Could you check a few things on this drawing? It's one solid part, dimensions in mm from its lowest x, y, z. A direction names the side the tool comes from. Give positions to 0.01 mm unless a question says otherwise; leave off trailing zeros. Loops run counter-clockwise (first coordinate to the right, second up) from the corner with the lowest first, then second, coordinate; pieces in that order, holes last.
1. Imagine slicing it at D-D (y = 10.25). List the corners of the cut face in (x, z) for me.
2. Imagine slicing it at B-B (x = 3). List the corners of the cut face in (y, z) for me, plus the area to 3 significant figures.
3. Imagine slicing it at C-C (z = 18). List the corners of the cut face in (x, y) for me, plus the area to 3 significant figures.
4. I need wall thicknesses on line 1 along X through (y, z) = (2.9, 3); line 2 along X through (y, z) = (3, 23); line 3 along X through (y, z) = (10.75, 15). Which ranges of each line are inside material? Lowest first, please.
5. Thinking about a two-plate mould opening in X: for the marked faces 1, 2 and 3, which applies, +X half, -X half, draft (parallel to the pull), parting line (faces both ways), or undercut?
6. For P1, Ø5.5, axis at x = 40.5, y = 3, coming from the +Z side; P2, Ø1.8, axis at x = 23, y = 9, coming from the -Z side; P3, Ø3.5, axis at y = 8, z = 28, coming from the +X side, each with a flat end and sliding along its axis, tell me the tip position at first contact or that it passes through.
7. For the marked faces 4 and 5, which set-ups out of +Z, -Z, +X, -X, +Y, -Y let a thin tool reach every point of the face, with its end or its side?
8. Imagine slicing it at A-A (z = 39). List the corners of the cut face in (x, y) for me.
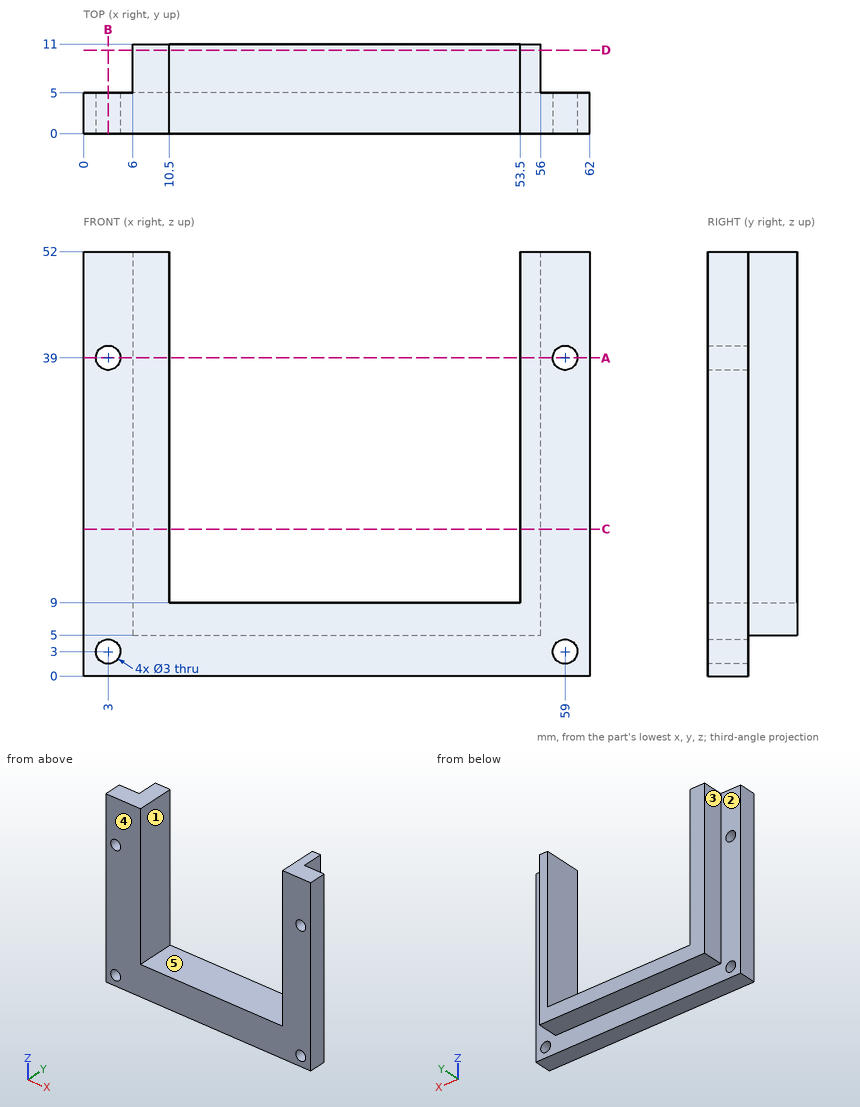
Derived:
1. outline: (6, 5) - (56, 5) - (56, 52) - (53.5, 52) - (53.5, 9) - (10.5, 9) - (10.5, 52) - (6, 52) - close
2. outline: (0, 0) - (5, 0) - (5, 1.5) - (0, 1.5) - close; (0, 4.5) - (5, 4.5) - (5, 37.5) - (0, 37.5) - close; (0, 40.5) - (5, 40.5) - (5, 52) - (0, 52) - close
2. area: 230 mm2
3. outline: (0, 0) - (10.5, 0) - (10.5, 11) - (6, 11) - (6, 5) - (0, 5) - close; (53.5, 0) - (62, 0) - (62, 5) - (56, 5) - (56, 11) - (53.5, 11) - close
3. area: 137 mm2
4. line 1: x = 0 to 1.5, 4.5 to 57.5, 60.5 to 62
4. line 2: x = 0 to 10.5, 53.5 to 62
4. line 3: x = 6 to 10.5, 53.5 to 56
5. face 1: undercut
5. face 2: draft
5. face 3: -X half
6. P1: stops at z = 9
6. P2: stops at z = 5
6. P3: stops at x = 56
7. face 4: +Z, -Z, +X, -X, -Y
7. face 5: +Z, +Y, -Y
8. outline: (0, 0) - (1.5, 0) - (1.5, 5) - (0, 5) - close; (4.5, 0) - (10.5, 0) - (10.5, 11) - (6, 11) - (6, 5) - (4.5, 5) - close; (53.5, 0) - (57.5, 0) - (57.5, 5) - (56, 5) - (56, 11) - (53.5, 11) - close; (60.5, 0) - (62, 0) - (62, 5) - (60.5, 5) - close
